Work out the finished part from the listing and answer in its coordinate system (mm). Face numbers are marked on the shaded views. A direction names the side the tool comes from. Coordinates: 2 decimals unless noted, no trailing zeros. Loops run counter-clockwise (first coordinate to the right, second up) from the corner with the lowest first, then second, coordinate; pieces in that order, holes last. Notation, with made-up numbers: (25.5, 52.25) -> (49.5, 52.25) arc R29 ccw to (49.5, 83.25) -> close; hole circle Ø4 at (-36.75, -13). An arc over 180 degrees is marked (long way). Use a Markdown table: item, result.
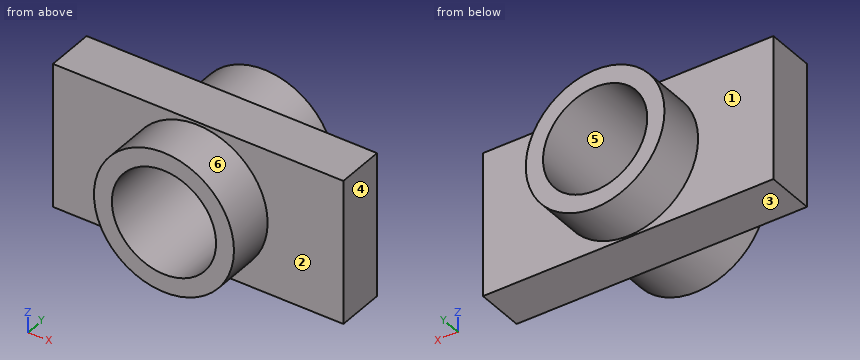
from build123d import *

# Parameters (mm, degrees)
F0_W     = 152.99622
F0_H     = 75.73466
F1_DEPTH = 25.4
F2_R     = 36.900045
F3_DEPTH = 25.4
F4_R     = 36.550704
F5_DEPTH = 25.4
F6_R     = 25.934616
F7_DEPTH = 25.4
F8_R     = 27.454989
F9_DEPTH = 83.312


with BuildPart() as f1:
    # F0 (on Front) → F1 (new body)
    with BuildSketch(Plane.XZ):
        with Locations((0.305381, 0.458073)):
            Rectangle(F0_W, F0_H)
    extrude(amount=F1_DEPTH)

    # F2 (on face) → F3 (join)
    with BuildSketch(Plane.XZ.offset(25.4)):
        Circle(F2_R)
    extrude(amount=F3_DEPTH)

    # F4 (on face) → F5 (join)
    with BuildSketch(Plane(origin=(0, 0, 0), x_dir=(-1, 0, 0), z_dir=(0, 1, 0))):
        Circle(F4_R)
    extrude(amount=F5_DEPTH)

    # F6 (on face) → F7 (cut)
    with BuildSketch(Plane.XZ.offset(50.8)):
        Circle(F6_R)
    extrude(amount=-F7_DEPTH, mode=Mode.SUBTRACT)

    # F8 (on face) → F9 (cut)
    with BuildSketch(Plane(origin=(0, 25.4, 0), x_dir=(-1, 0, 0), z_dir=(0, 1, 0))):
        Circle(F8_R)
    extrude(amount=-F9_DEPTH, mode=Mode.SUBTRACT)


solid = f1.part
Q1. For the marked faces 1, 2 and 3, determine the directions among +Z, -Z, +X, -X, +Y, -Y from which every point of the face is accessible in a straight line to the end or side of a thin tool.
Solved:
| item | result |
|---|---|
| face 1 | +Y |
| face 2 | -Y |
| face 3 | -Z, +X, -X, +Y, -Y |
Q2. Section A-A on z = 0 is taken. Determine the outline of the cut face in (x, y).
Solved:
| item | result |
|---|---|
| outline | (-76.19, -25.4) -> (-36.9, -25.4) -> (-36.9, -50.8) -> (-27.45, -50.8) -> (-27.45, 25.4) -> (-36.55, 25.4) -> (-36.55, 0) -> (-76.19, 0) -> close; (27.45, -50.8) -> (36.9, -50.8) -> (36.9, -25.4) -> (76.8, -25.4) -> (76.8, 0) -> (36.55, 0) -> (36.55, 25.4) -> (27.45, 25.4) -> close |
Q3. Section D-D on z = 30.5 is taken. Determine the outline of the cut face in (x, y), and give its area (3 significant figures).
Solved:
| item | result |
|---|---|
| outline | (-76.19, -25.4) -> (-20.77, -25.4) -> (-20.77, -50.8) -> (20.77, -50.8) -> (20.77, -25.4) -> (76.8, -25.4) -> (76.8, 0) -> (20.14, 0) -> (20.14, 25.4) -> (-20.14, 25.4) -> (-20.14, 0) -> (-76.19, 0) -> close |
| area | 5,960 mm² |
Q4. Section C-C on y = -8 is taken. Determine the outline of the cut face in (x, z), and give its area (3 significant figures).
Solved:
| item | result |
|---|---|
| outline | (-76.19, -37.41) -> (76.8, -37.41) -> (76.8, 38.33) -> (-76.19, 38.33) -> close; hole circle Ø54.91 at (0, 0) |
| area | 9,220 mm² |
Q5. Determine the mould class of the marked faces 4, 5 and 6 for opening direction X: pulls with the +X half, pulls with the -X half, needs draft (parallel to the pull), parting line crosses it, or undercut.
Solved:
| item | result |
|---|---|
| face 4 | pulls with the +X half |
| face 5 | undercut |
| face 6 | parting line crosses it |
Q6. Section B-B on x = 0 is taken. Determine the outline of the cut face in (y, z).
Solved:
| item | result |
|---|---|
| outline | (-50.8, -36.9) -> (-25.4, -36.9) -> (-25.4, -37.41) -> (0, -37.41) -> (0, -36.55) -> (25.4, -36.55) -> (25.4, -27.45) -> (-50.8, -27.45) -> close; (-50.8, 27.45) -> (25.4, 27.45) -> (25.4, 36.55) -> (0, 36.55) -> (0, 38.33) -> (-25.4, 38.33) -> (-25.4, 36.9) -> (-50.8, 36.9) -> close |
Q7. Given pin 1 Ø1 at (x, y) = (27, 10) entering from +Z; pin 2 Ø12 at (x, z) = (-53, -23.5) entering from -Y; pin 3 Ø8 at (x, y) = (-32, -38) entering from -Z, each flat-ended and moving along its own axis, determine where each tip first touches the part or whether it passes through.
Solved:
| item | result |
|---|---|
| pin 1 | z = 25.17 |
| pin 2 | y = -25.4 |
| pin 3 | z = -24.03 |
Q8. Consider line 1 (Z direction, x = 0, y = -25); line 2 (Z direction, x = 0, y = -26); line 3 (Y direction, x = 41, z = 33). Determine where each line is inside the solid, lowest interval first. Write a range as [from, to].
Solved:
| item | result |
|---|---|
| line 1 | [-37.41, -27.45], [27.45, 38.33] |
| line 2 | [-36.9, -27.45], [27.45, 36.9] |
| line 3 | [-25.4, 0] |
